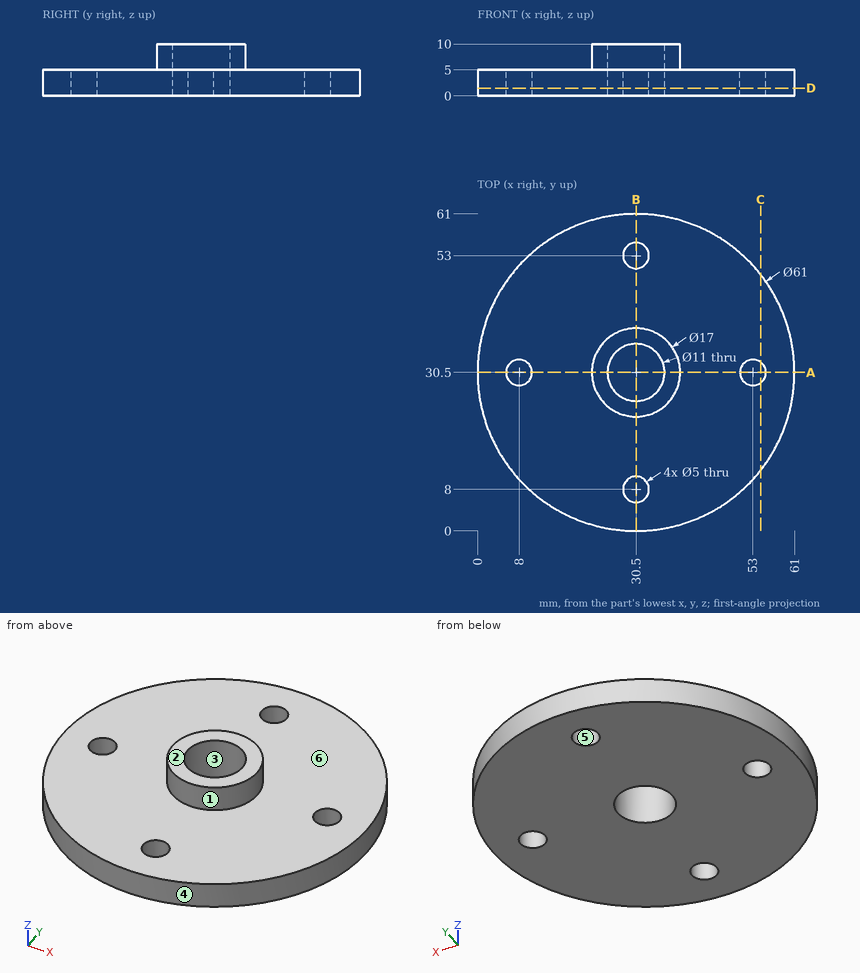
Print and shaded views of the part. All mm, measured from the part's lowest x, y and z. A direction names the side the tool comes from. Give positions to 0.01 mm unless a question says otherwise; leave off trailing zeros. Write each loop counter-clockwise with the first axis right and the second up, starting at its lowest first coordinate (ties: lowest second). Pieces come first, ordered by that corner, then holes. Notation, with made-up numbers: (-32.75, -38.5) - (11.25, -38.5) arc R30 ccw to (11.25, -9.5) - close; hole circle Ø7 at (89.5, 74.25). An arc over 180 degrees is marked (long way). One line per question, with ' | ' between items. Start each with the question number.
(1) Slice it at C-C on x = 54.5. Write the cut outline in (y, z).
(2) Slice it at A-A on y = 30.5. Write the cut outline in (x, z).
(3) Pin check, flat tips, straight feed: P1, Ø6, axis at y = 13, z = 5, coming from the -X side; P2, Ø5, axis at y = 47, z = 9, coming from the +X side; P3, Ø6, axis at x = 51, z = 5.5, coming from the -Y side; P4, Ø1.5, axis at x = 42.5, y = 22.5, coming from the +Z side. Stop position of each tip, or through.
(4) Wall check: line 1 along Y through (x, z) = (30.5, 2.7); line 2 along Y through (x, z) = (30.5, 6.5); line 3 along Z through (x, y) = (30, 39.5). Give the ranges that are in metal, low to high. Write a range as from..to.
(5) 3-axis set-ups, long thin cutter, end or side, ignore diameter. For the marked faces 1 and 2: which of +Z, -Z, +X, -X, +Y, -Y reach the whole face in a straight line?
(6) Two-plate mould, pull along X, no slides. Class the marked faces 3, 4, 5 and 6: +X half, -X half, draft (parallel to the pull), parting line (faces both ways), or undercut.
(7) Slice it at D-D on z = 1.5. Write the cut outline in (x, y).
Results below:
1) outline: (11.68, 0) - (28.5, 0) - (28.5, 5) - (11.68, 5) - close; (32.5, 0) - (49.32, 0) - (49.32, 5) - (32.5, 5) - close
2) outline: (0, 0) - (5.5, 0) - (5.5, 5) - (0, 5) - close; (10.5, 0) - (25, 0) - (25, 10) - (22, 10) - (22, 5) - (10.5, 5) - close; (36, 0) - (50.5, 0) - (50.5, 5) - (39, 5) - (39, 10) - (36, 10) - close; (55.5, 0) - (61, 0) - (61, 5) - (55.5, 5) - close
3) P1: x = 3.67 | P2: through | P3: y = 5.55 | P4: z = 5
4) line 1: 0..5.5, 10.5..25, 36..50.5, 55.5..61 | line 2: 22..25, 36..39 | line 3: 0..5
5) face 1: +Z | face 2: +Z, +X, -X, +Y, -Y
6) face 3: undercut | face 4: parting line | face 5: undercut | face 6: draft
7) outline: circle Ø61 at (30.5, 30.5); hole circle Ø5 at (8, 30.5); hole circle Ø11 at (30.5, 30.5); hole circle Ø5 at (30.5, 8); hole circle Ø5 at (30.5, 53); hole circle Ø5 at (53, 30.5)
